Read the model definition and answer for the solid it produces. Units are mm, in the model's axes. A direction names the side the tool comes from. Round coordinates to 2 decimals unless told otherwise and drop trailing zeros. Order: outer loops, then holes, each group sorted by start corner. A loop starts at its lowest first (then second) coordinate and runs counter-clockwise, first axis right, second up. Notation, with made-up numbers: (77.5, 18.5) - (100.5, 18.5) arc R27 cw to (100.5, 50.5) - close; hole circle Ø3 at (87, 55.25). An arc over 180 degrees is marked (long way). Answer as a JSON object with one key per item and string values. Group by question number.
Q1. A cutting plane is placed at A-A on y = -4.75. Count the separate pieces of the cut face and the enclosed holes in it, and give its area (3 significant figures).
Q2. A tool of negligible diameter and unlimited length cuts with its end or side. For faces 4 (the flat face through (0, -6, -4)), 5 (the cylindrical face through (-0.69, -1.57, -3.1)), from which of +Z, -Z, +X, -X, +Y, -Y can it reach the whole face along a straight path? Write none if from no direction.
Q3. A cutting plane is placed at D-D on z = 2.75. Determine the outline of the cut face in (x, y) (3 decimals), and give its area (3 significant figures).
Q4. Consider line 1 (Z direction, x = 0, y = -3) (3 decimals); line 2 (Z direction, x = 2, y = -2.5); line 3 (Y direction, x = -3.5, z = -3.5) (3 decimals). Determine where each line is inside the solid, lowest interval first.
Q5. Given pin 1 Ø3 at (x, z) = (1, -1.5) entering from -Y (3 decimals); pin 2 Ø5 at (x, y) = (-3.5, -6) entering from +Z; pin 3 Ø5 at (x, z) = (0, 0) entering from +Y; pin 4 Ø0.6 at (y, z) = (-7, -4.5) entering from +X, each flat-ended and moving along its own axis, determine where each tip first touches the part or whether it passes through.
Q6. The mould has two halves that part along Z. Classify faces 1 (the cylindrical face through (-1.707, -3.131, 12.329)), 2 (the flat face through (3, -6.35, 12)), 3 (the cylindrical face through (0, -3, 16)): pulls with the +Z half, pulls with the -Z half, needs draft (parallel to the pull), parting line crosses it, or undercut.
Q7. A cutting plane is placed at B-B on y = -6.75. Determine the outline of the cut face in (x, z).
```python
from build123d import *

# Parameters (mm, degrees)
F0_R     = 6.35
F0_R_2   = 3.175
F1_DEPTH = 3.175
F2_R     = 6.35
F2_R_2   = 5.0165
F3_DEPTH = 6.35
F4_R     = 3.175
F5_DEPTH = 6.35
F7_DEPTH = 6.35
F8_R     = 0.3048


# Not quite as in the source:
# - a feature names something its author has since deleted; it is built from what else it names


with BuildPart() as f1:
    # F0 (on Front) → F1 (new body)
    with BuildSketch(Plane.XZ):
        Circle(F0_R)
        Circle(F0_R_2, mode=Mode.SUBTRACT)
    extrude(amount=F1_DEPTH)

    # F2 (on face) → F3 (join)
    with BuildSketch(Plane.XZ.offset(3.175)):
        Circle(F2_R)
        Circle(F2_R_2, mode=Mode.SUBTRACT)
    extrude(amount=F3_DEPTH)

    # F4 (on face) → F5 (join)
    with BuildSketch(Plane(origin=(0, 0, 0), x_dir=(-1, 0, 0), z_dir=(0, 1, 0))):
        with BuildLine():
            ThreePointArc((-6.35, 9.652), (-5.7675394704, 6.9953125029), (-4.1270115096, 4.826))
            ThreePointArc((-4.1270115096, 4.826), (0, 6.35), (4.1270115096, 4.826))
            ThreePointArc((4.1270115096, 4.826), (5.7675394704, 6.9953125029), (6.35, 9.652))
            ThreePointArc((6.35, 9.652), (0, 16.002), (-6.35, 9.652))
        make_face()
        with Locations((0, 9.652)):
            Circle(F4_R, mode=Mode.SUBTRACT)
        with BuildLine():
            Line((-6.35, 9.652), (-6.35, 0))
            ThreePointArc((-6.35, 0), (-5.7675394704, 2.6566874971), (-4.1270115096, 4.826))
            ThreePointArc((-4.1270115096, 4.826), (-5.7675394704, 6.9953125029), (-6.35, 9.652))
        make_face()
        with BuildLine():
            ThreePointArc((4.1270115096, 4.826), (5.7675394704, 2.6566874971), (6.35, 0))
            Line((6.35, 0), (6.35, 9.652))
            ThreePointArc((6.35, 9.652), (5.7675394704, 6.9953125029), (4.1270115096, 4.826))
        make_face()
    extrude(amount=-F5_DEPTH)

    # F6 (on face) → F7 (join, through all)
    with BuildSketch(Plane.XZ.offset(9.525)):
        with BuildLine():
            Line((-1.1049, -4.0005), (-1.1049, -4.8933085167))
            ThreePointArc((-1.1049, -4.8933085167), (0, -5.0165), (1.1049, -4.8933085167))
            Line((1.1049, -4.8933085167), (1.1049, -4.0005))
            Line((1.1049, -4.0005), (-1.1049, -4.0005))
        make_face()
    extrude(amount=-F7_DEPTH)

    # F8
    f8_edges = [f1.edges().sort_by_distance(p)[0] for p in [
        (1.1049, -6.35, -4.0005),
        (-1.1049, -6.35, -4.0005),
    ]]
    fillet(f8_edges, radius=F8_R)


solid = f1.part
```
Result set:
{
 "1": {"separate pieces": "1", "enclosed holes": "2", "area": "141 mm²"},
 "2": {"face 4": "-Y", "face 5": "+Y, -Y"},
 "3": {"outline": "(-6.35, -6.35) - (-5.724, -6.35) - (-5.724, -9.525) - (-4.196, -9.525) - (-4.196, -3.175) - (-1.587, -3.175) - (-1.587, 0) - (-6.35, 0) - close; (1.587, -3.175) - (4.196, -3.175) - (4.196, -9.525) - (5.724, -9.525) - (5.724, -6.35) - (6.35, -6.35) - (6.35, 0) - (1.587, 0) - close", "area": "53.6 mm²"},
 "4": {"line 1": "z = -6.35 to -3.175, 3.175 to 6.477, 12.827 to 16.002", "line 2": "z = -6.03 to -2.47, 2.47 to 7.19, 12.12 to 15.68", "line 3": "y = -3.175 to 0"},
 "5": {"pin 1": "stops at y = -3.175", "pin 2": "stops at z = 15.92", "pin 3": "passes through", "pin 4": "stops at x = 4.76"},
 "6": {"face 1": "undercut", "face 2": "needs draft", "face 3": "pulls with the +Z half"},
 "7": {"outline": "circle Ø12.7 at (0, 0); hole (-1.1, -4.89) - (-1.1, -4.31) arc R0.3 cw to (-0.8, -4) - (0.8, -4) arc R0.3 cw to (1.1, -4.31) - (1.1, -4.89) arc R5.02 ccw (long way) to start"}
}
